Could you check a few things on this model? Use its own coordinates, in mm. A direction names the side the tool comes from. Give positions to 0.01 mm unless a question says otherwise; leave off trailing zeros. Loops run counter-clockwise (first coordinate to the right, second up) from the corner with the lowest first, then second, coordinate; pieces in that order, holes last. Notation, with made-up numbers: M -15,46.5 L 13,46.5 A22 ccw 13,68.5 Z; hole C 82.25,14 d2. An arc over 180 degrees is marked long. Use a Markdown table: item, result. Add a question column.
1) Suppose I cut it at A-A on z = 6. List the corners of the cut face in (x, y) for me.
2) Which directions (+Z, -Z, +X, -X, +Y, -Y) give clear straight access to the entire face, cutting with the end or side of a thin tool? Please do faces 1 (the flat face through (25, -1, 5.2)), 2 (the flat face through (10, 0, 6.4)), 3 (the flat face through (17, 3.75, 2)).
3) Suppose I cut it at D-D on y = 6.75. List the corners of the cut face in (x, z) for me, and give its area (3 significant figures).
4) Suppose I cut it at C-C on z = 1.25. List the corners of the cut face in (x, y) for me, and give its area (3 significant figures).
5) We'd pull the mould along X, two halves only. Please class faces 4 (the cylindrical face through (-6.81, -6.83, 3.16)), 5 (the flat face through (15, 9.75, 3)), 6 (the cylindrical face through (8.5, 6, 3.2)): +X half, -X half, draft (parallel to the pull), parting line (faces both ways), or undercut.
6) Suppose I cut it at B-B on x = 9.5. Count the separate pieces of the cut face and the enclosed holes in it, and give its area (3 significant figures).
7) If I drill on line 1 along Y through (x, z) = (9.5, 4.25); line 2 along X through (y, z) = (6, 3.5); line 3 along Y through (x, z) = (9.5, 3.5), over which ranges is the centre line in solid material (lowest first)? Write a range as [from, to].
8) Will these pins go through, and if not, where does the flat tip stop? pin 1 Ø3 at (x, y) = (0, 0) entering from -Z; pin 2 Ø1 at (x, z) = (-1, 5.5) entering from +Y.
```python
from build123d import *

# Parameters (mm, degrees)
SKETCH1_R           = 1.25
BOSS_EXTRUDE4_DEPTH = 4
FILLET1_R           = 10
SKETCH2_R           = 1.25
BOSS_EXTRUDE5_DEPTH = 1.2
SKETCH3_R           = 3
SKETCH3_R_2         = 1.25
BOSS_EXTRUDE6_DEPTH = 1.2


with BuildPart() as part:
    # Sketch1 → Boss-Extrude4 (new body)
    with BuildSketch(Plane.XY):
        Polygon((-9.75, 9.75), (-9.75, 0), (-9.75, -9.75), (29.5, -9.75), (29.5, -6.75), (29.5, 6.75), (29.5, 9.75), align=None)
        with Locations((9.5, -6.75)):
            Circle(SKETCH1_R, mode=Mode.SUBTRACT)
        with Locations((9.5, 6.75)):
            Circle(SKETCH1_R, mode=Mode.SUBTRACT)
        with BuildLine():
            ThreePointArc((4.901044183, -6.003521127), (-3.322604971, -7.001628111), (-7.75, 0))
            ThreePointArc((-7.75, 0), (-3.322604971, 7.001628111), (4.901044183, 6.003521127))
            ThreePointArc((4.901044183, 6.003521127), (7.868246727, 4.330212616), (11.22497216, 3.75))
            Line((11.22497216, 3.75), (23.75, 3.75))
            ThreePointArc((23.75, 3.75), (26.401650429, 2.651650429), (27.5, 0))
            ThreePointArc((27.5, 0), (26.401650429, -2.651650429), (23.75, -3.75))
            Line((23.75, -3.75), (11.22497216, -3.75))
            ThreePointArc((11.22497216, -3.75), (7.868246727, -4.330212616), (4.901044183, -6.003521127))
        make_face(mode=Mode.SUBTRACT)
    extrude(amount=BOSS_EXTRUDE4_DEPTH)

    # Fillet1
    # the kernel refuses this fillet: 10 mm, written as the material it takes off along each edge
    with BuildSketch(Plane(origin=(-9.75, -9.75, -25), x_dir=(0, 1, 0), z_dir=(0, 0, 1))) as fillet1_piece_1:
        with BuildLine():
            CenterArc((FILLET1_R, -FILLET1_R), FILLET1_R, 90, 90)
            Line((0, -FILLET1_R), (0, 0))
            Line((0, 0), (FILLET1_R, 0))
        make_face()
    extrude(amount=54, mode=Mode.SUBTRACT)
    with BuildSketch(Plane(origin=(-9.75, 9.75, -25), x_dir=(0, -1, 0), z_dir=(0, 0, 1))) as fillet1_piece_2:
        with BuildLine():
            CenterArc((FILLET1_R, FILLET1_R), FILLET1_R, 180, 90)
            Line((0, FILLET1_R), (0, 0))
            Line((0, 0), (FILLET1_R, 0))
        make_face()
    extrude(amount=54, mode=Mode.SUBTRACT)

    # Sketch2 → Boss-Extrude5 (add)
    # profile 1 of 4: a face of its own
    with BuildSketch(Plane.XY.offset(4)):
        with BuildLine():
            ThreePointArc((8.882472313, 4.028236041), (5.388428188, 8.129565896), (0.25, 9.75))
            ThreePointArc((0.25, 9.75), (-6.732120022, 6.908910532), (-9.746874512, 0))
            ThreePointArc((-9.746874512, 0), (-6.957195545, -6.682267477), (-0.388423062, -9.729599992))
            Line((-0.388423062, -9.729599992), (0.667724562, -9.730320853))
            ThreePointArc((0.667724562, -9.730320853), (5.561475334, -8.012177738), (8.882472313, -4.028236041))
            ThreePointArc((8.882472313, -4.028236041), (6.780629621, -4.791885277), (4.901044183, -6.003521127))
            ThreePointArc((4.901044183, -6.003521127), (-7.75, 0), (4.901044183, 6.003521127))
            ThreePointArc((4.901044183, 6.003521127), (6.780629621, 4.791885277), (8.882472313, 4.028236041))
        make_face()
    # profile 2 of 4: a face of its own
    with BuildSketch(Plane.XY.offset(4)):
        with BuildLine():
            ThreePointArc((9.753204602, 0), (9.5330365, 2.060634631), (8.882472313, 4.028236041))
            ThreePointArc((8.882472313, 4.028236041), (6.780629621, 4.791885277), (4.901044183, 6.003521127))
            ThreePointArc((4.901044183, 6.003521127), (-7.75, 0), (4.901044183, -6.003521127))
            ThreePointArc((4.901044183, -6.003521127), (6.780629621, -4.791885277), (8.882472313, -4.028236041))
            ThreePointArc((8.882472313, -4.028236041), (9.5330365, -2.060634631), (9.753204602, 0))
        make_face()
        Circle(SKETCH2_R, mode=Mode.SUBTRACT)
    # profile 3 of 4: a face of its own
    with BuildSketch(Plane.XY.offset(4)):
        with BuildLine():
            Line((29.5, -9.75), (29.5, 9.75))
            Line((29.5, 9.75), (0.25, 9.75))
            ThreePointArc((0.25, 9.75), (5.388428188, 8.129565896), (8.882472313, 4.028236041))
            ThreePointArc((8.882472313, 4.028236041), (10.045489135, 3.819802631), (11.22497216, 3.75))
            Line((11.22497216, 3.75), (23.75, 3.75))
            ThreePointArc((23.75, 3.75), (27.5, 0), (23.75, -3.75))
            Line((23.75, -3.75), (11.22497216, -3.75))
            ThreePointArc((11.22497216, -3.75), (10.045489135, -3.819802631), (8.882472313, -4.028236041))
            ThreePointArc((8.882472313, -4.028236041), (5.561475334, -8.012177738), (0.667724562, -9.730320853))
            Line((0.667724562, -9.730320853), (29.5, -9.75))
        make_face()
        with Locations((9.5, -6.75)):
            Circle(SKETCH2_R, mode=Mode.SUBTRACT)
        with Locations((9.5, 6.75)):
            Circle(SKETCH2_R, mode=Mode.SUBTRACT)
    # profile 4 of 4: a face of its own
    with BuildSketch(Plane.XY.offset(4)):
        with BuildLine():
            ThreePointArc((11.22497216, 3.75), (10.045489135, 3.819802631), (8.882472313, 4.028236041))
            ThreePointArc((8.882472313, 4.028236041), (9.5330365, 2.060634631), (9.753204602, 0))
            ThreePointArc((9.753204602, 0), (9.5330365, -2.060634631), (8.882472313, -4.028236041))
            ThreePointArc((8.882472313, -4.028236041), (10.045489135, -3.819802631), (11.22497216, -3.75))
            Line((11.22497216, -3.75), (23.75, -3.75))
            ThreePointArc((23.75, -3.75), (27.5, 0), (23.75, 3.75))
            Line((23.75, 3.75), (11.22497216, 3.75))
        make_face()
        with Locations((23.75, 0)):
            Circle(SKETCH2_R, mode=Mode.SUBTRACT)
    extrude(amount=BOSS_EXTRUDE5_DEPTH)

    # Sketch3 → Boss-Extrude6 (add)
    # profile 1 of 2: a face of its own
    with BuildSketch(Plane.XY.offset(5.2)):
        with BuildLine():
            ThreePointArc((9.75, 0), (6.938066581, 6.850235917), (0.124208797, 9.749208797))
            ThreePointArc((0.124208797, 9.749208797), (-6.777009203, 6.864853594), (-9.746874512, 0))
            ThreePointArc((-9.746874512, 0), (-6.957195545, -6.682267477), (-0.388423062, -9.729599992))
            Line((-0.388423062, -9.729599992), (0.619672772, -9.730288056))
            ThreePointArc((0.619672772, -9.730288056), (7.110003851, -6.671607395), (9.75, 0))
        make_face()
        Circle(SKETCH3_R, mode=Mode.SUBTRACT)
    # profile 2 of 2: a face of its own
    with BuildSketch(Plane.XY.offset(5.2)):
        with BuildLine():
            Line((29.5, 9.75), (0.25, 9.75))
            ThreePointArc((0.25, 9.75), (0.187103155, 9.749802197), (0.124208797, 9.749208797))
            ThreePointArc((0.124208797, 9.749208797), (6.938066581, 6.850235917), (9.75, 0))
            ThreePointArc((9.75, 0), (7.110003851, -6.671607395), (0.619672772, -9.730288056))
            Line((0.619672772, -9.730288056), (29.5, -9.75))
            Line((29.5, -9.75), (29.5, 9.75))
        make_face()
        with Locations((9.5, -6.75)):
            Circle(SKETCH3_R_2, mode=Mode.SUBTRACT)
        with Locations((9.5, 6.75)):
            Circle(SKETCH3_R_2, mode=Mode.SUBTRACT)
        with Locations((23.75, 0)):
            Circle(SKETCH3_R, mode=Mode.SUBTRACT)
    extrude(amount=BOSS_EXTRUDE6_DEPTH)


solid = part.part
```
Answer block:
| question | item | result |
|---|---|---|
| 1 | outline | M -9.75,0 A10 ccw -0.39,-9.73 L 29.5,-9.75 L 29.5,9.75 L 0.25,9.75 A10 ccw 0.12,9.75 A10 ccw Z; hole C 0,0 d6; hole C 9.5,-6.75 d2.5; hole C 9.5,6.75 d2.5; hole C 23.75,0 d6 |
| 2 | face 1 | +Z |
| 2 | face 2 | +Z, +X, -X, +Y, -Y |
| 2 | face 3 | -Z |
| 3 | outline | M -6.89,0 L -3.81,0 L -3.81,4 L 3.81,4 L 3.81,0 L 8.25,0 L 8.25,6.4 L -6.89,6.4 Z; M 10.75,0 L 29.5,0 L 29.5,6.4 L 10.75,6.4 Z |
| 3 | area | 186 mm^2 |
| 4 | outline | M -9.75,0 A10 ccw 0.25,-9.75 L 29.5,-9.75 L 29.5,9.75 L 0.25,9.75 A10 ccw Z; hole M 4.9,-6 A10 cw 11.22,-3.75 L 23.75,-3.75 A3.75 ccw 23.75,3.75 L 11.22,3.75 A10 cw 4.9,6 A7.75 ccw long Z; hole C 9.5,-6.75 d2.5; hole C 9.5,6.75 d2.5 |
| 4 | area | 375 mm^2 |
| 5 | face 4 | -X half |
| 5 | face 5 | draft |
| 5 | face 6 | undercut |
| 6 | separate pieces | 3 |
| 6 | enclosed holes | 0 |
| 6 | area | 61.6 mm^2 |
| 7 | line 1 | y = [-9.74, -8], [-5.5, 5.5], [8, 9.75] |
| 7 | line 2 | x = [-7.56, -4.91], [4.91, 8.5], [10.5, 29.5] |
| 7 | line 3 | y = [-9.75, -8], [-5.5, -3.9], [3.9, 5.5], [8, 9.75] |
| 8 | pin 1 | stops at z = 4 |
| 8 | pin 2 | stops at y = 9.72 |
